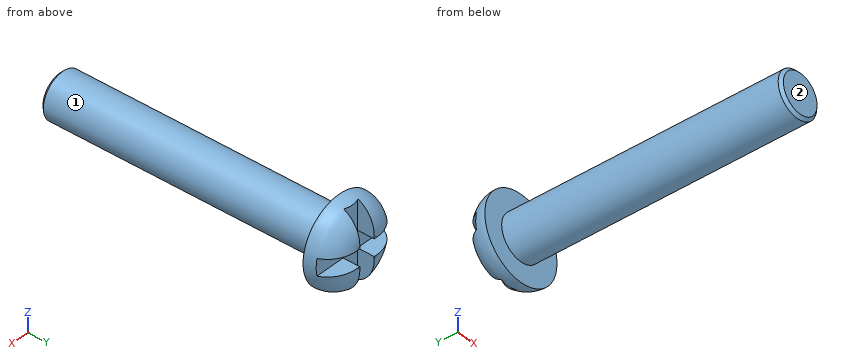
Autodesk Inventor part; units mm, degrees
ref_plane "YZ Plane" through (0, 0, 0) normal (1, 0, 0) x (0, 1, 0)
ref_plane "XZ Plane" through (0, 0, 0) normal (0, 1, 0) x (-1, 0, 0)
ref_plane "XY Plane" through (0, 0, 0) normal (0, 0, 1) x (1, 0, 0)
sketch "Sketch1" plane through (0, 0, 0) normal (0, 1, 0) x (-1, 0, 0)
  circle A0 centre (0, 0) radius 4
  dimension "d0" = 8
extrude "Extrusion1" add sketch "Sketch1" along normal blind 50
sketch "Sketch2" plane through (0, 50, 0) normal (0, 1, 0) x (1, 0, 0)
  circle A0 centre (0, 0) radius 7.5
  dimension "d3" = 15
extrude "Extrusion2" add sketch "Sketch2" along normal blind 5
fillet "Fillet1" radius 5 1 edges at (-7.5, 55, 0)
sketch "Sketch3" plane through (0, 55, 0) normal (0, 1, 0) x (1, 0, 0)
  line L0 (7.4391, -1.5) -> (-7.4391, -1.5)
  line L1 (-7.4391, -1.5) -> (-7.4391, 1.5)
  line L2 (-7.4391, 1.5) -> (7.4391, 1.5)
  line L3 (7.4391, 1.5) -> (7.4391, -1.5)
  line L4 (7.4391, -1.5) -> (-7.4391, 1.5) construction
  line L5 (-7.4391, -1.5) -> (7.4391, 1.5) construction
  line L6 (1.5, -6.8733) -> (-1.5, -6.8733)
  line L7 (-1.5, -6.8733) -> (-1.5, 6.8733)
  line L8 (-1.5, 6.8733) -> (1.5, 6.8733)
  line L9 (1.5, 6.8733) -> (1.5, -6.8733)
  line L10 (1.5, -6.8733) -> (-1.5, 6.8733) construction
  line L11 (-1.5, -6.8733) -> (1.5, 6.8733) construction
  point P0 (0, 0)
  dimension "d7" = 3
  dimension "d8" = 3
extrude "Extrusion3" cut sketch "Sketch3" against normal blind 3
thread "Thread1"
chamfer "Chamfer1" distance 0.5 angle 45 1 edges at (4, 0, 0)
properties part number "Vijs"
Source: CAD feature listing. Evaluate the final solid. Frame: model axes, mm. Face numbers are marked on the shaded views. A direction names the side the tool comes from. Round coordinates to 2 decimals unless told otherwise and drop trailing zeros. Loops run counter-clockwise (first coordinate to the right, second up) from the corner with the lowest first, then second, coordinate; pieces in that order, holes last. Notation, with made-up numbers: M 70.5,8 L 122.5,8 A21 ccw 122.5,17 Z; hole C 7,5 d3. An arc over 180 degrees is marked long. Use a Markdown table: item, result. Add a question column.
1. Set-up query: the marked faces 1 and 2. Return all of +Z, -Z, +X, -X, +Y, -Y with unobstructed straight access to the full face (end or side cutting, diameter ignored); none if empty.
2. Cut plane A-A, the plane y = 29.5. Output: boundary loops of the cut face in (x, z).
3. Ray query, line 1 along Z through (x, y) = (0, 18); line 2 along Y through (x, z) = (-0.75, -1.5); line 3 along X through (y, z) = (5, 0.25). Return the intervals inside material, ascending. Write a range as [from, to].
4. Contact query for flat-ended pins moving along their axis: pin 1 (2.5 mm diameter, centred on y = 54, z = -5, fed in from -X); pin 2 (6 mm diameter, centred on x = 0.5, y = 11, fed in from +Z); pin 3 (8 mm diameter, centred on y = 12.5, z = 5.5, fed in from +X). Output: stop coordinate, or through.
Solution:
| question | item | result |
|---|---|---|
| 1 | face 1 | -Y |
| 1 | face 2 | +Z, -Z, +X, -X, -Y |
| 2 | outline | C 0,0 d8 |
| 3 | line 1 | z = [-4, 4] |
| 3 | line 2 | y = [0, 52] |
| 3 | line 3 | x = [-3.99, 3.99] |
| 4 | pin 1 | stops at x = -4.92 |
| 4 | pin 2 | stops at z = 4 |
| 4 | pin 3 | stops at x = 3.71 |
